Could you check a few things on this drawing? It's one solid part, dimensions in mm from its lowest x, y, z. A direction names the side the tool comes from. Round coordinates to 2 decimals unless told otherwise and drop trailing zeros. Write each loop counter-clockwise with the first axis right and the second up, starting at its lowest first coordinate (ties: lowest second). Pieces come first, ordered by that corner, then holes. Notation, with made-up numbers: M 28,-32.5 L 61,-32.5 A20 cw 61,-2.5 Z; hole C 5,58.25 d6. An arc over 180 degrees is marked long. One line per item, written item: value. Start each with the question number.
(1) I want a section at A-A on z = 3. Please give me the cut outline in (x, y), and give its area (3 significant figures).
(2) Which directions (+Z, -Z, +X, -X, +Y, -Y) give clear straight access to the entire face, cutting with the end or side of a thin tool? Please do the marked faces 1, 2 and 3.
(3) I want a section at C-C on y = 19. Please give me the cut outline in (x, z).
(4) I want a section at D-D on y = 5.75. Please give me the cut outline in (x, z) (1 decimal).
(5) If I drill on L1, parallel to Z at x = 6, y = 18.6; L2, parallel to Y at x = 3.75, z = 15; L3, parallel to X at y = 18.5, z = 18, over which ranges is the centre line in solid material (lowest first)?
(6) I want a section at B-B on x = 6. Please give me the cut outline in (y, z) (1 decimal).
(7) Thinking about a two-plate mould opening in X: for the marked faces 4, 5 and 6, which applies, released by +X, released by -X, zero draft, split by the parting line, or undercut?
(8) I'm going to push flat-ended pins straight in: pin 1 Ø1.5 at (x, y) = (6.5, 6.5) entering from +Z; pin 2 Ø5 at (y, z) = (8, 29) entering from -X; pin 3 Ø3 at (x, z) = (3.5, 7.5) entering from -Y; pin 4 Ø1.5 at (x, z) = (4, 37) entering from +Y. Where does each tip first touch, or does it pass through?
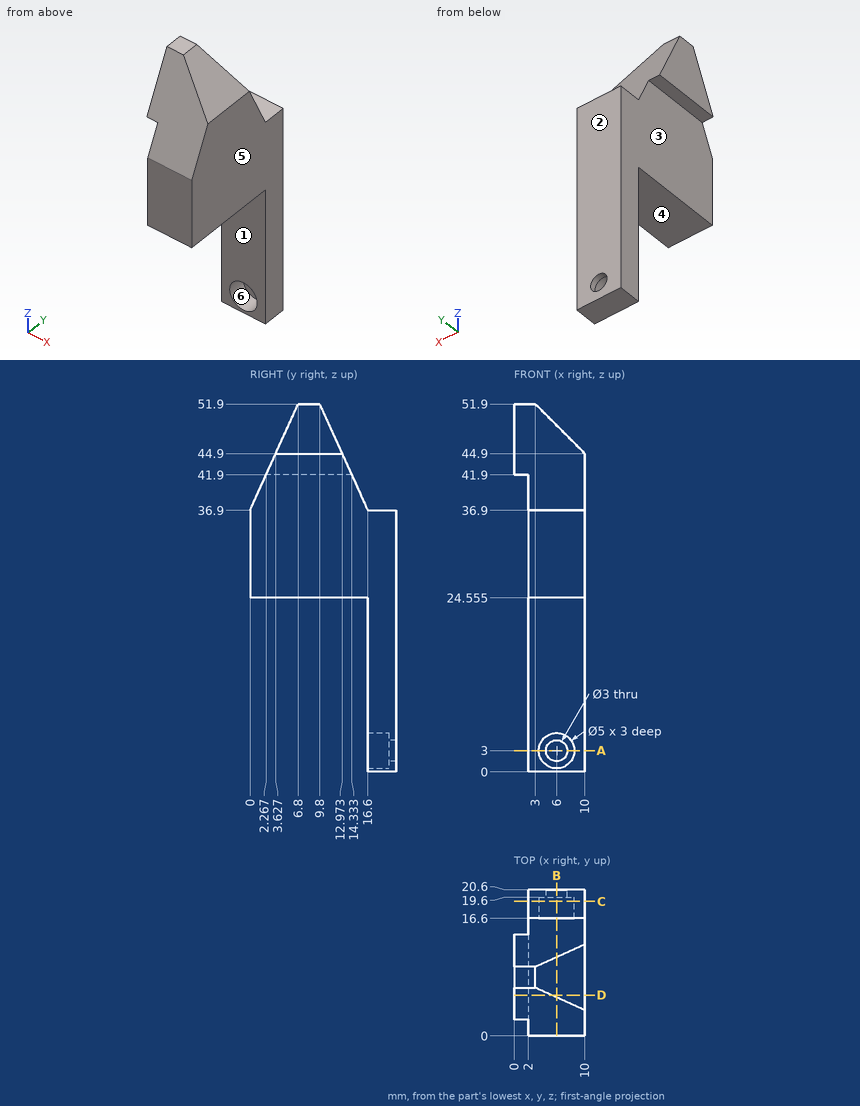
Found:
1. outline: M 2,16.6 L 3.5,16.6 L 3.5,19.6 L 4.5,19.6 L 4.5,20.6 L 2,20.6 Z; M 7.5,19.6 L 8.5,19.6 L 8.5,16.6 L 10,16.6 L 10,20.6 L 7.5,20.6 Z
1. area: 14.0 mm²
2. face 1: -Z, +X, -X, -Y
2. face 2: +Z, -Z, +X, -X, +Y
2. face 3: -Z, -X, +Y, -Y
3. outline: M 2,0 L 10,0 L 10,36.9 L 2,36.9 Z; hole C 6,3 d5
4. outline: M 0,41.9 L 2,41.9 L 2,24.6 L 10,24.6 L 10,44.9 L 5.3,49.6 L 0,49.6 Z
5. L1: z = 0 to 0.5, 5.5 to 36.9
5. L2: y = 16.6 to 20.6
5. L3: x = 2 to 10
6. outline: M 0,24.6 L 16.6,24.6 L 16.6,5.5 L 19.6,5.5 L 19.6,4.5 L 20.6,4.5 L 20.6,36.9 L 16.6,36.9 L 11.2,48.9 L 5.4,48.9 L 0,36.9 Z; M 16.6,0 L 20.6,0 L 20.6,1.5 L 19.6,1.5 L 19.6,0.5 L 16.6,0.5 Z
7. face 4: zero draft
7. face 5: released by +X
7. face 6: undercut
8. pin 1: stops at z = 49.15
8. pin 2: stops at x = 2
8. pin 3: stops at y = 16.6
8. pin 4: stops at y = 20.6
